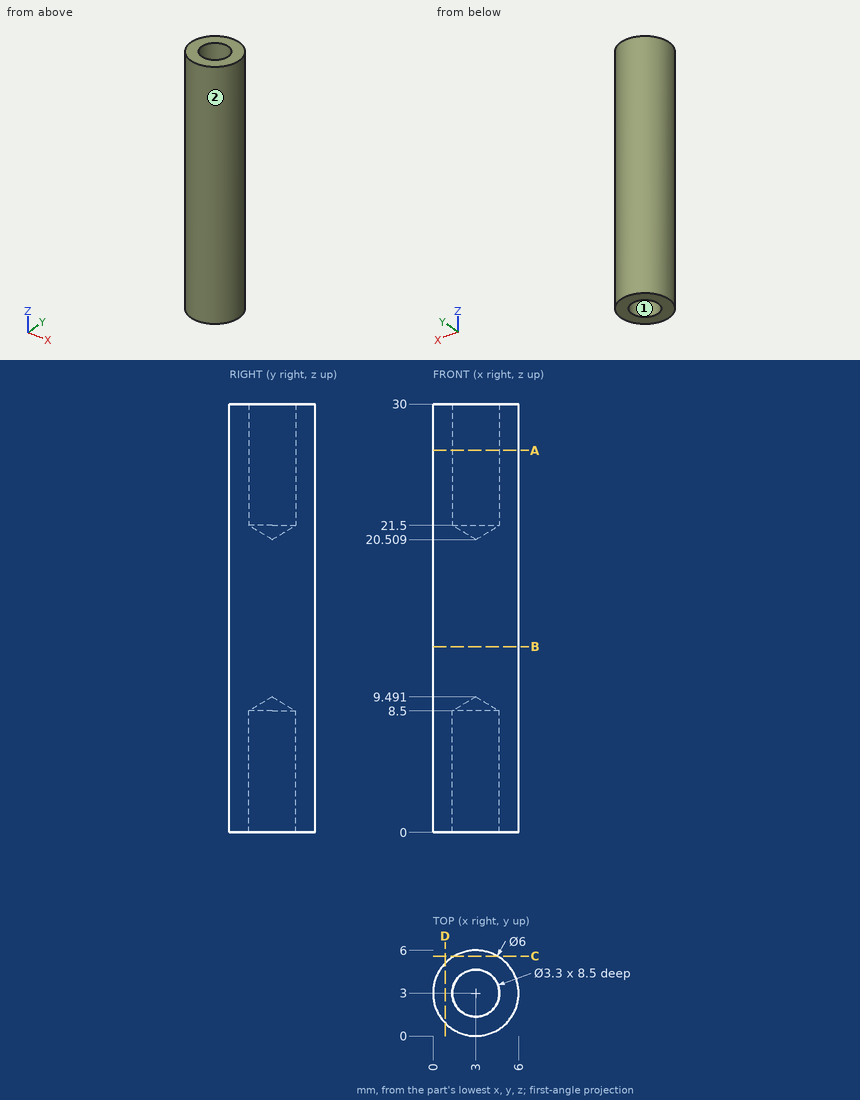
Here's the drawing with two shaded views (mm, measured from the low corner). I have some questions. Coordinates: 2 decimals unless noted, no trailing zeros. Order: outer loops, then holes, each group sorted by start corner. A loop starts at its lowest first (then second) coordinate and runs counter-clockwise, first axis right, second up.
Item 1: I need wall thicknesses on line 1 (Y direction, x = 3, z = 23.75); line 2 (X direction, y = 3.7, z = 28) (1 decimal). Which ranges of each line are inside material? Lowest first, please.
Result sheet:
line 1: y = 0 to 1.35, 4.65 to 6
line 2: x = 0.1 to 1.5, 4.5 to 5.9
Item 2: If we section it at A-A on z = 26.75: List the corners of the cut face in (x, y) for me, plus the area to 3 significant figures.
Result sheet:
outline: circle Ø6 at (3, 3); hole circle Ø3.3 at (3, 3)
area: 19.7 mm2
Item 3: If we section it at B-B on z = 13: List the corners of the cut face in (x, y) for me.
Result sheet:
outline: circle Ø6 at (3, 3)
Item 4: If we section it at C-C on y = 5.6: List the corners of the cut face in (x, z) for me.
Result sheet:
outline: (1.5, 0) - (4.5, 0) - (4.5, 30) - (1.5, 30) - close
Item 5: If we mould it in two halves opening along X, with no side actions, what happens to the marked faces 1 and 2? For each: +X half, -X half, draft (parallel to the pull), parting line (faces both ways), or undercut.
Result sheet:
face 1: undercut
face 2: parting line
Item 6: If we section it at D-D on x = 0.85: List the corners of the cut face in (y, z) for me.
Result sheet:
outline: (0.91, 0) - (5.09, 0) - (5.09, 30) - (0.91, 30) - close
Item 7: For P1, Ø2, axis at x = 3, y = 3, coming from the -Z side; P2, Ø1, axis at y = 1.5, z = 10.5, coming from the +X side, each with a flat end and sliding along its axis, tell me the tip position at first contact or that it passes through.
Result sheet:
P1: stops at z = 8.89
P2: stops at x = 5.83
